Work out the finished part from the listing and answer in its coordinate system (mm). A direction names the side the tool comes from. Give positions to 0.01 mm unless a question says otherwise; leave off trailing zeros. Order: outer loops, then holes, each group sorted by start corner. A loop starts at its lowest first (then second) coordinate and runs counter-clockwise, first axis right, second up. Notation, with made-up numbers: M 40.5,49 L 85.5,49 A31 cw 85.5,73 Z; hole C 56,21.25 d1. An arc over 180 degrees is marked long. One line per item, written item: value.
from build123d import *

# Parameters (mm, degrees)
F0_W     = 300
F0_H     = 200
F0_W_2   = 295
F0_H_2   = 195
F0_W_3   = 290
F0_H_3   = 190
F1_DEPTH = 10
F2_DEPTH = 3
F3_DEPTH = 3
F4_R     = 5
F5_R     = 5


with BuildPart() as f1:
    # F0 (on Top) → F1 (new body)
    with BuildSketch(Plane.XY):
        Rectangle(F0_W, F0_H)
        Rectangle(F0_W_2, F0_H_2, mode=Mode.SUBTRACT)
        Rectangle(F0_W_2, F0_H_2)
        Rectangle(F0_W_3, F0_H_3, mode=Mode.SUBTRACT)
    extrude(amount=F1_DEPTH)

    # F0 (on Top) → F2 (cut)
    with BuildSketch(Plane.XY):
        Rectangle(F0_W_2, F0_H_2)
        Rectangle(F0_W_3, F0_H_3, mode=Mode.SUBTRACT)
    extrude(amount=F2_DEPTH, mode=Mode.SUBTRACT)

    # F0 (on Top) → F3 (join)
    with BuildSketch(Plane.XY):
        Rectangle(F0_W_2, F0_H_2)
        Rectangle(F0_W_3, F0_H_3, mode=Mode.SUBTRACT)
        Rectangle(F0_W_3, F0_H_3)
    extrude(amount=F3_DEPTH)

    # F4
    f4_edges = [f1.edges().sort_by_distance(p)[0] for p in [
        (-150, -100, 5),
        (150, -100, 5),
        (150, 100, 5),
        (-150, 100, 5),
    ]]
    fillet(f4_edges, radius=F4_R)

    # F5
    f5_edges = [f1.edges().sort_by_distance(p)[0] for p in [
        (150, 0, 0),
        (148.535534, -98.535534, 0),
        (148.535534, 98.535534, 0),
        (0, -100, 0),
        (0, 100, 0),
        (-148.535534, -98.535534, 0),
        (-148.535534, 98.535534, 0),
        (-150, 0, 0),
    ]]
    fillet(f5_edges, radius=F5_R)


solid = f1.part
(1) Section B-B, the plane x = -42.5 is taken. Give the vertices of the cut face in (y, z), then the cut area to 3 significant figures.
Findings:
outline: M -100,5 A5 ccw -95,0 L 95,0 A5 ccw 100,5 L 100,10 L 95,10 L 95,3 L -95,3 L -95,10 L -100,10 Z
area: 659 mm^2
(2) Section C-C, the plane y = 18.5 is taken. Give the vertices of the cut face in (x, z), then the cut area to 3 significant figures.
Findings:
outline: M -150,5 A5 ccw -145,0 L 145,0 A5 ccw 150,5 L 150,10 L 145,10 L 145,3 L -145,3 L -145,10 L -150,10 Z
area: 959 mm^2
(3) Given P1, Ø1.5, axis at y = -47.5, z = 4.5, coming from the +X side; P2, Ø2, axis at x = -20.5, z = 1.5, coming from the -Y side; P3, Ø1, axis at y = -20.5, z = 1.5, coming from the +X side, each flat-ended and moving along its own axis, determine where each tip first touches the part or whether it passes through.
Findings:
P1: stops at x = 150
P2: stops at y = -99.33
P3: stops at x = 149
(4) Section A-A, the plane z = 7.25 is taken. Give the vertices of the cut face in (x, y).
Findings:
outline: M -150,-95 A5 ccw -145,-100 L 145,-100 A5 ccw 150,-95 L 150,95 A5 ccw 145,100 L -145,100 A5 ccw -150,95 Z; hole M -145,-95 L 145,-95 L 145,95 L -145,95 Z
(5) Determine the mould class of faces 3 (the flat face through (-45, -96, 10)), 4 (the flat face through (-145, -1, 6)) for opening direction Y: pulls with the +Y half, pulls with the -Y half, needs draft (parallel to the pull), parting line crosses it, or undercut.
Findings:
face 3: needs draft
face 4: undercut
(6) Find the intervals of material crossed by probe 1 along X at (y, z) = (49.5, 5.75); probe 2 along Y at (x, z) = (27, 6.5); probe 3 along Z at (x, y) = (55.5, -66), in increasing order. Write a range as from..to.
Findings:
probe 1: x = -150..-145, 145..150
probe 2: y = -100..-95, 95..100
probe 3: z = 0..3
(7) Which of the six approach directions +Z, -Z, +X, -X, +Y, -Y give full straight-line access (tool end or side, diameter ignored) to faces 1 (the flat face through (145, -1, 6)), 2 (the flat face through (-2, 1, 0))?
Findings:
face 1: +Z
face 2: -Z, +X, -X, +Y, -Y
